```python
from build123d import *

# Parameters (mm, degrees)
PAD002_DEPTH    = 7
PAD003_DEPTH    = 3
CHAMFER003_SIZE = 1.5
SKETCH019_W     = 4
SKETCH019_H     = 8.5
POCKET003_DEPTH = 7.001
SKETCH020_W     = 4
SKETCH020_H     = 8.5
POCKET004_DEPTH = 4
SKETCH024_W     = 11.6
SKETCH024_H     = 2.9
PAD006_DEPTH    = 16.9
SKETCH025_W     = 11.6
SKETCH025_H     = 2.8
PAD007_DEPTH    = 1.9
CHAMFER005_SIZE = 1.5
SKETCH026_W     = 6.8
SKETCH026_H     = 10.4
PAD008_DEPTH    = 3.2
SKETCH034_W     = 10
SKETCH034_H     = 30
PAD014_DEPTH    = 0.2


with BuildPart() as part:
    # Sketch006 → Pad002 (new body)
    with BuildSketch(Plane.XY.offset(4)):
        Polygon((-62, 2.5), (-62, -16), (62, -16), (62, 2.5), (42, 2.5), (31.5, -8), (-31.5, -8), (-42, 2.5), align=None)
    extrude(amount=PAD002_DEPTH)

    # Sketch007 (on Face9 of Pad002) → Pad003 (join)
    with BuildSketch(Plane(origin=(0, 0, 4), x_dir=(1, 0, 0), z_dir=(0, 0, -1))):
        with BuildLine():
            Line((-31.5, 8), (31.5, 8))
            Line((37.293259, 2.206741), (31.5, 8))
            Line((38.566051, 3.479533), (37.293259, 2.206741))
            Line((32.772792, 9.272792), (38.566051, 3.479533))
            ThreePointArc((32.772792, 9.272792), (32.18883, 9.662983), (31.5, 9.8))
            Line((31.5, 9.8), (-31.5, 9.8))
            ThreePointArc((-31.5, 9.8), (-32.18883, 9.662983), (-32.772792, 9.272792))
            Line((-38.566051, 3.479533), (-32.772792, 9.272792))
            Line((-37.293259, 2.206741), (-38.566051, 3.479533))
            Line((-31.5, 8), (-37.293259, 2.206741))
        make_face()
    extrude(amount=PAD003_DEPTH)

    # Chamfer003
    chamfer003_edges = [part.edges().sort_by_distance(p)[0] for p in [
        (-35.669422, -6.376163, 4),
    ]]
    chamfer(chamfer003_edges, length=CHAMFER003_SIZE)

    # Sketch019 (on Face1 of Chamfer003) → Pocket003 (cut, through all)
    with BuildSketch(Plane(origin=(0, 0, 4), x_dir=(1, 0, 0), z_dir=(0, 0, -1))):
        with Locations((-60, 6.75)):
            Rectangle(SKETCH019_W, SKETCH019_H)
        with Locations((60, 6.75)):
            Rectangle(SKETCH019_W, SKETCH019_H)
    extrude(amount=-POCKET003_DEPTH, mode=Mode.SUBTRACT)

    # Sketch020 (on Face31 of Pocket003) → Pocket004 (cut)
    with BuildSketch(Plane.XY.offset(11)):
        with Locations((-56, -6.75)):
            Rectangle(SKETCH020_W, SKETCH020_H)
        with Locations((56, -6.75)):
            Rectangle(SKETCH020_W, SKETCH020_H)
    extrude(amount=-POCKET004_DEPTH, mode=Mode.SUBTRACT)

    # Sketch024 (on Face27 of Pocket004) → Pad006 (join)
    with BuildSketch(Plane.XY.offset(11)):
        with Locations((0, -7.45)):
            Rectangle(SKETCH024_W, SKETCH024_H)
    extrude(amount=-PAD006_DEPTH)

    # Sketch025 (on Face37 of Pad006) → Pad007 (join)
    with BuildSketch(Plane.XZ.offset(8.9)):
        with Locations((0, -4.5)):
            Rectangle(SKETCH025_W, SKETCH025_H)
    extrude(amount=PAD007_DEPTH)

    # Chamfer005
    chamfer005_edges = [part.edges().sort_by_distance(p)[0] for p in [
        (0, -10.8, -5.9),
        (-5.8, -10.8, -4.5),
        (5.8, -10.8, -4.5),
    ]]
    chamfer(chamfer005_edges, length=CHAMFER005_SIZE)

    # Sketch026 (on Face37 of Chamfer005) → Pad008 (join)
    with BuildSketch(Plane(origin=(0, 0, 4), x_dir=(1, 0, 0), z_dir=(0, 0, -1))):
        with Locations((-46.5, 2.7)):
            Rectangle(SKETCH026_W, SKETCH026_H)
        with Locations((46.5, 2.7)):
            Rectangle(SKETCH026_W, SKETCH026_H)
    extrude(amount=PAD008_DEPTH)

    # Sketch034 (on Face12 of Pad008) → Pad014 (join)
    with BuildSketch(Plane.XY.offset(11)):
        with Locations((-61, -7)):
            Rectangle(SKETCH034_W, SKETCH034_H)
        with Locations((61, -7)):
            Rectangle(SKETCH034_W, SKETCH034_H)
    extrude(amount=-PAD014_DEPTH)


solid = part.part
```
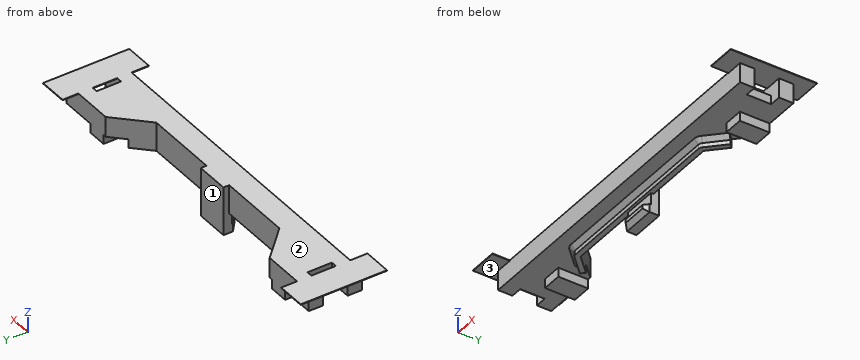
Could you check a few things on this model? Use its own coordinates, in mm. Face numbers are marked on the shaded views. Give positions to 0.01 mm unless a question says otherwise; leave off trailing zeros. Loops run counter-clockwise (first coordinate to the right, second up) from the corner with the lowest first, then second, coordinate; pieces in that order, holes last. Notation, with made-up numbers: (-12.75, 76.5) - (7.25, 76.5) arc R25 cw to (7.25, 114.5) - close; hole circle Ø5 at (49, 67.25). An arc over 180 degrees is marked (long way). Use one line per item in the form item = value.
1. I want a section at B-B (z = 8.5). Please give me the cut outline in (x, y).
Response values:
outline = (-62, -16) - (62, -16) - (62, -11) - (54, -11) - (54, -2.5) - (62, -2.5) - (62, 2.5) - (42, 2.5) - (31.5, -8) - (5.8, -8) - (5.8, -6) - (-5.8, -6) - (-5.8, -8) - (-31.5, -8) - (-42, 2.5) - (-62, 2.5) - (-62, -2.5) - (-54, -2.5) - (-54, -11) - (-62, -11) - close
2. I need wall thicknesses on probe 1 along X at (y, z) = (-0.5, 2.75); probe 2 along Z at (x, y) = (36, -13.5); probe 3 along Y at (x, z) = (8, 5.25). Which ranges of each line are inside material? Lowest first, please.
Response values:
probe_1 = -49.9 to -43.1, 43.1 to 49.9
probe_2 = 4 to 11
probe_3 = -16 to -8
3. I want a section at D-D (y = -13.5). Please give me the cut outline in (x, z).
Response values:
outline = (-66, 10.8) - (-62, 10.8) - (-62, 4) - (62, 4) - (62, 10.8) - (66, 10.8) - (66, 11) - (-66, 11) - close
4. I want a section at A-A (y = -0.5). Please give me the cut outline in (x, z).
Response values:
outline = (-66, 10.8) - (-62, 10.8) - (-62, 4) - (-49.9, 4) - (-49.9, 0.8) - (-43.1, 0.8) - (-43.1, 4) - (-39, 4) - (-39, 11) - (-66, 11) - close; (39, 4) - (43.1, 4) - (43.1, 0.8) - (49.9, 0.8) - (49.9, 4) - (62, 4) - (62, 10.8) - (66, 10.8) - (66, 11) - (39, 11) - close
5. Thinking about a two-plate mould opening in Y: for the marked faces 1, 2 and 3, which applies, released by +Y, released by -Y, zero draft, split by the parting line, or undercut?
Response values:
face_1 = released by +Y
face_2 = zero draft
face_3 = undercut
6. I want a section at C-C (x = -26). Please give me the cut outline in (y, z).
Response values:
outline = (-16, 4) - (-11.3, 4) - (-9.8, 2.5) - (-9.8, 1) - (-8, 1) - (-8, 11) - (-16, 11) - close
7. I'm going to push flat-ended pins straight in: pin 1 Ø10 at (x, y) = (-4.5, -13) entering from -Z; pin 2 Ø3.5 at (x, y) = (-45, -0.5) entering from -Z; pin 3 Ø3.5 at (x, z) = (47, 2.5) entering from -Y; pin 4 Ø3.5 at (y, z) = (-8, 5) entering from +X. Where does each tip first touch, or does it pass through?
Response values:
pin_1 = -5.9
pin_2 = 0.8
pin_3 = -16
pin_4 = 58
